```python
from build123d import *

# Parameters (mm, degrees)
CROQUIS1_R              = 9.5
CROQUIS1_R_2            = 6
SALIENTE_EXTRUIR1_DEPTH = 6
MATRIZC1_COUNT          = 3
CHAFL_N1_SIZE           = 0.5
CHAFL_N2_SIZE           = 0.5


with BuildPart() as part:
    # Croquis1 → Saliente-Extruir1 (new body)
    with BuildSketch(Plane(origin=(0, 0, 0), x_dir=(1, 0, 0), z_dir=(0, 1, 0))):
        with Locations(Location((0, 0, 0), (0, 0, 270))):
            Circle(CROQUIS1_R)
        with Locations(Location((0, 0, 0), (0, 0, 270))):
            Circle(CROQUIS1_R_2, mode=Mode.SUBTRACT)
    extrude(amount=SALIENTE_EXTRUIR1_DEPTH)

    # Croquis3 → Taladro roscado M31 (revolve, cut)
    with BuildSketch(Plane(origin=(0, 3, 9.5), x_dir=(0, -1, 0), z_dir=(1, 0, 0))):
        Polygon((0, 0), (0, 9.251075774), (1.25, 8.5), (1.25, 0), align=None)
    taladro_roscado_m31 = revolve(axis=Axis((0, 3, 15.85), (0, 0, -1)), mode=Mode.SUBTRACT)

    # MatrizC1: Taladro roscado M31 ×3 about axis
    matrizc1_axis = Axis((0, 0, 0), (0, 1, 0))
    for i in range(1, MATRIZC1_COUNT):
        add(taladro_roscado_m31.rotate(matrizc1_axis, i * 360 / MATRIZC1_COUNT), mode=Mode.SUBTRACT)

    # Chaflán1
    chafl_n1_edges = [part.edges().sort_by_distance(p)[0] for p in [
        (0, 0, -6),
        (0, 6, -6),
    ]]
    chamfer(chafl_n1_edges, length=CHAFL_N1_SIZE)

    # Chaflán2
    chafl_n2_edges = [part.edges().sort_by_distance(p)[0] for p in [
        (0, 0, -9.5),
        (0, 6, -9.5),
    ]]
    chamfer(chafl_n2_edges, length=CHAFL_N2_SIZE)


solid = part.part
```
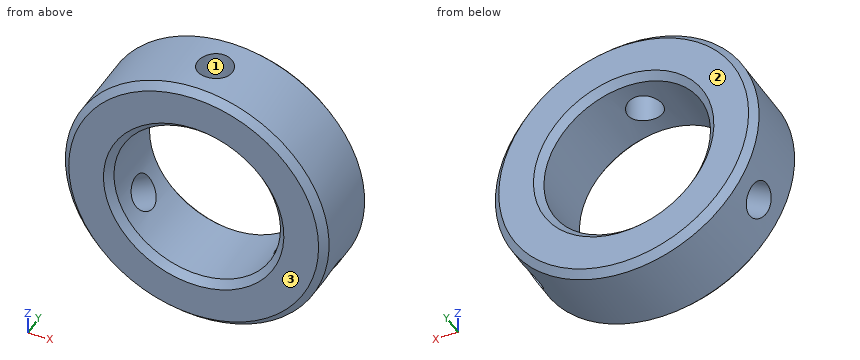
Geometry check sheet. Reference: the model listing, model coordinates, mm. Face numbers are marked on the shaded views. Coordinates: 2 decimals unless noted, no trailing zeros. Write each loop counter-clockwise with the first axis right and the second up, starting at its lowest first coordinate (ties: lowest second). Pieces come first, ordered by that corner, then holes. Notation, with made-up numbers: M 21.25,-22.5 L 52.25,-22.5 A25 ccw 52.25,12.5 Z; hole C -12.5,-4 d11. An arc over 180 degrees is marked long. One line per item, written item: value. Start each with the question number.
(1) Sectioned sample at A-A, the plane x = 0. Enter the section's corners in (y, z), and give its area (4 significant figures).
(2) Scan lines: line 1 along X through (y, z) = (4, 0); line 2 along X through (y, z) = (3, 8.5); line 3 along Z through (x, y) = (-4, 4.8). Record each from-to range of solid material in increasing order. Write a range as [from, to].
(3) Sectioned sample at D-D, the plane y = 1.15. Enter the section's corners in (x, z), and give its area (3 significant figures).
(4) Depth check by flat-ended pin: pin 1 (8 mm diameter, centred on x = -6, z = 0.5, fed in from +Y); pin 2 (1 mm diameter, centred on x = 3, y = 3, fed in from -Z); pin 3 (1 mm diameter, centred on x = 2.5, z = 5, fed in from +Y); pin 4 (2 mm diameter, centred on x = 0, y = 3, fed in from +Z). Enter the tip coordinate at first touch or a pass-through.
(5) Sectioned sample at B-B, the plane z = 0. Enter the section's corners in (x, y).
(6) Release check for a two-part mould opening along Y. For the marked faces 1, 2 and 3 record: released by +Y, released by -Y, zero draft, split by the parting line, or undercut.
(7) Sectioned sample at C-C, the plane y = 2.6. Enter the section's corners in (x, z).
Filled sheet:
1. outline: M 0,-9 L 0.5,-9.5 L 5.5,-9.5 L 6,-9 L 6,-6.5 L 5.5,-6 L 0.5,-6 L 0,-6.5 Z; M 0,6.5 L 0.5,6 L 1.75,6 L 1.75,9.5 L 0.5,9.5 L 0,9 Z; M 4.25,6 L 5.5,6 L 6,6.5 L 6,9 L 5.5,9.5 L 4.25,9.5 Z
1. area: 32.25 mm²
2. line 1: [-9.5, -6], [6, 9.5]
2. line 2: [-4.24, -1.25], [1.25, 4.24]
2. line 3: [-8.62, -4.47], [4.47, 8.62]
3. outline: C 0,0 d19; hole C 0,0 d12
3. area: 170 mm²
4. pin 1: y = 6
4. pin 2: z = -9.17
4. pin 3: y = 5.59
4. pin 4: z = -5.92
5. outline: M -9.5,0.5 L -9,0 L -6.5,0 L -6,0.5 L -6,5.5 L -6.5,6 L -9,6 L -9.5,5.5 Z; M 6,0.5 L 6.5,0 L 9,0 L 9.5,0.5 L 9.5,5.5 L 9,6 L 6.5,6 L 6,5.5 Z
6. face 1: undercut
6. face 2: released by +Y
6. face 3: released by -Y
7. outline: M -8.76,-3.69 L -5.69,-1.92 A6 cw -1.18,5.88 L -1.18,9.43 A9.5 ccw Z; M -7.57,-5.74 A9.5 ccw 7.57,-5.74 L 4.5,-3.97 A6 cw -4.5,-3.97 Z; M 1.18,5.88 A6 cw 5.69,-1.92 L 8.76,-3.69 A9.5 ccw 1.18,9.43 Z
